```python
from build123d import *

# Parameters (mm, degrees)
LEVER_DEPTH      = 1.8
LEVER_DEPTH_BACK = 1.8
CUT_DEPTH        = 15.439772455
FILLET_1_R       = 0.5


with BuildPart() as part:
    # Эскиз1 → Lever (new, two sides: drawn at the far end of the back side and taken through both)
    with BuildSketch(Plane(origin=(2.85, 0, 0), x_dir=(0, 0, -1), z_dir=(1, 0, 0)).offset(-LEVER_DEPTH_BACK)):
        with BuildLine():
            Line((5.55, 4.85), (5.55, 6.042820323))
            ThreePointArc((5.55, 6.042820323), (5.440072487, 6.355619708), (5.158626179, 6.530878059))
            Line((5.158626179, 6.530878059), (-12.45, 10.45))
            Line((-12.45, 10.45), (-12.417412146, 10.596417321))
            Line((-12.417412146, 10.596417321), (5.191214033, 6.677295379))
            ThreePointArc((5.191214033, 6.677295379), (5.557094233, 6.449459523), (5.7, 6.042820323))
            Line((5.7, 6.042820323), (5.7, 4.85))
            Line((5.7, 4.85), (5.55, 4.85))
        make_face()
    extrude(amount=LEVER_DEPTH + LEVER_DEPTH_BACK)

    # Эскиз2 → Cut (cut, through all)
    with BuildSketch(Plane(origin=(0, 4.95, 0), x_dir=(1, 0, 0), z_dir=(0, 1, 0))):
        Polygon((1.05, 5.8), (1.35, -12.45), (1.05, -12.45), align=None)
        Polygon((4.65, 5.8), (4.65, -12.45), (4.35, -12.45), align=None)
        with BuildLine():
            Line((2.35, 5.8), (3.35, 5.8))
            Line((3.35, 5.8), (3.20551955, -1.905624011))
            ThreePointArc((3.20551955, -1.905624011), (3.115706509, -2.11411119), (2.90557227, -2.2))
            Line((2.90557227, -2.2), (2.79442773, -2.2))
            ThreePointArc((2.79442773, -2.2), (2.584293491, -2.11411119), (2.49448045, -1.905624011))
            Line((2.49448045, -1.905624011), (2.35, 5.8))
        make_face()
    extrude(amount=CUT_DEPTH, mode=Mode.SUBTRACT)

    # Скругление1
    fillet_1_edges = [part.edges().sort_by_distance(p)[0] for p in [
        (4.350267845, 10.52320866, 12.433706073),
        (1.349732155, 10.52320866, 12.433706073),
    ]]
    fillet(fillet_1_edges, radius=FILLET_1_R)


solid = part.part
```
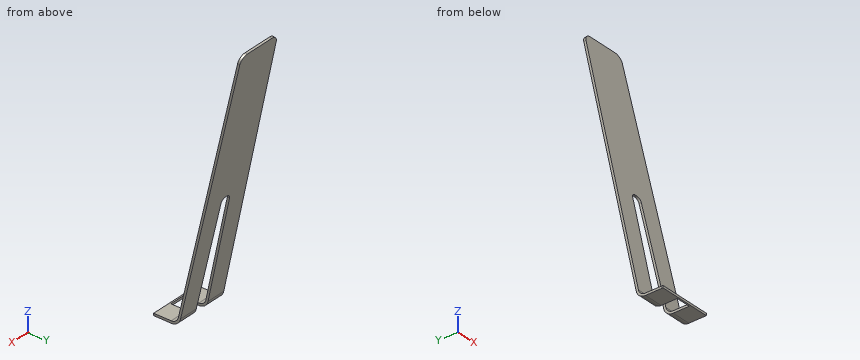
The listing builds one solid part. Answer for the finished solid, in the listing's coordinates (mm). Coordinates: 2 decimals unless noted, no trailing zeros. Write each loop counter-clockwise with the first axis right and the second up, starting at its lowest first coordinate (ties: lowest second). Pieces come first, ordered by that corner, then holes.
Q1. Section C-C, the plane y = 5.45 is taken. Write down the section's boundary in (x, z), then the cut area to 3 significant figures.
Returned:
outline: (1.05, -5.7) - (2.35, -5.7) - (2.35, -5.55) - (1.05, -5.55) - close; (3.35, -5.7) - (4.65, -5.7) - (4.65, -5.55) - (3.35, -5.55) - close
area: 0.390 mm2
Q2. Given P1, Ø2, axis at x = 3, z = 7.5, coming from the -Y side; P2, Ø1.3, axis at x = 3, y = 5.5, coming from the +Z side, each flat-ended and moving along its own axis, determine where each tip first touches the part or whether it passes through.
Returned:
P1: stops at y = 9.13
P2: stops at z = -5.55
Q3. Find the intervals of material crossed by line 1 along Y through (x, z) = (2.15, 11.75); line 2 along Y through (x, z) = (3.95, 3.5); line 3 along Z through (x, y) = (2.1, 5.4), in increasing order.
Returned:
line 1: y = 10.29 to 10.45
line 2: y = 8.46 to 8.61
line 3: z = -5.7 to -5.55
Q4. Section B-B, the plane x = 2.05 is taken. Write down the section's boundary in (y, z).
Returned:
outline: (4.85, -5.7) - (6.04, -5.7) arc R0.65 ccw to (6.68, -5.19) - (10.6, 12.42) - (10.45, 12.45) - (6.53, -5.16) arc R0.5 cw to (6.04, -5.55) - (4.85, -5.55) - close
Q5. Section D-D, the plane z = 4 is taken. Write down the section's boundary in (x, y), then the cut area to 3 significant figures.
Returned:
outline: (1.21, 8.57) - (4.49, 8.57) - (4.49, 8.72) - (1.21, 8.72) - close
area: 0.504 mm2
Q6. Section A-A, the plane z = 1.75 is taken. Write down the section's boundary in (x, y).
Returned:
outline: (1.17, 8.07) - (2.49, 8.07) - (2.49, 8.22) - (1.17, 8.22) - close; (3.21, 8.07) - (4.53, 8.07) - (4.53, 8.22) - (3.21, 8.22) - close
